Source: CAD feature listing. Evaluate the final solid. Frame: model axes, mm. A direction names the side the tool comes from. Coordinates: 2 decimals unless noted, no trailing zeros. Order: outer loops, then holes, each group sorted by start corner. A loop starts at its lowest first (then second) coordinate and runs counter-clockwise, first axis right, second up. Notation, with made-up numbers: (74.25, 67.25) -> (117.25, 67.25) arc R25 ccw to (117.25, 104.25) -> close; hole circle Ø10 at (34.5, -29.75). An arc over 180 degrees is marked (long way). Write item = value, one per line. Start each with the question number.
Item 1: Mould query, pull axis X, two halves, no side actions, for faces 1 (the cylindrical face through (-0.09, -37.1, 2.03)), 2 (the flat face through (0, 40, 2)), 3 (the flat face through (0, 6.66, 2.92)). Classes: released by +X, released by -X, zero draft, split by the parting line, or undercut.
Item 2: Set-up query: faces 4 (the flat face through (5, -10, 2)), 5 (the flat face through (-5, 1, 0)). Return all of +Z, -Z, +X, -X, +Y, -Y with unobstructed straight access to the full face (end or side cutting, diameter ignored); none if empty.
Item 3: Section query C-C (x = 4.25). Output: boundary loops of the cut face in (y, z), then the cut area to 3 significant figures.
Item 4: Section query B-B (y = 7.3). Output: boundary loops of the cut face in (x, z).
Item 5: Contact query for flat-ended pins moving along their axis: pin 1 (2 mm diameter, centred on y = -7.5, z = 2, fed in from +X); pin 2 (4 mm diameter, centred on x = 0, y = 35, fed in from -Z). Output: stop coordinate, or through.
Item 6: Section query D-D (y = -9). Output: boundary loops of the cut face in (x, z), then the cut area to 3 significant figures.
Item 7: Ray query, line 1 along Z through (x, y) = (-7.5, 7.3); line 2 along X through (y, z) = (-35, 1.55); line 3 along Y through (x, z) = (-5.5, 2.15). Return the intervals inside material, ascending. Write a range as [from, to].
Item 8: Section query A-A (z = 2). Output: boundary loops of the cut face in (x, y).
Solid Edge part; units mm, degrees
sketch "Sketch1" plane through (0, 0, 0) normal (0, 0, 1) x (1, 0, 0)
  line L0 (-10, -40) -> (10, -40)
  line L1 (10, -40) -> (10, 40)
  line L2 (10, 40) -> (-10, 40)
  line L3 (-10, 40) -> (-10, -40)
  circle A0 centre (0, 0) radius 4.6
  dimension "D1" = 10
  dimension "D2" = 10
extrude "Protrusion1" add sketch "Sketch1" along normal blind 4
sketch "Sketch2" plane through (0, 0, 4) normal (0, 0, 1) x (1, 0, 0)
  line L0 (0, 10) -> (10, 10)
  line L1 (10, 10) -> (10, -10)
  line L2 (10, -10) -> (0, -10)
  line L3 (0, -10) -> (0, 10)
  dimension "D1" = 10
extrude "Cutout1" cut sketch "Sketch2" against normal up to next
sketch "Sketch3" plane through (0, 0, 4) normal (0, 0, 1) x (0, 1, 0)
  circle A0 centre (35, 0) radius 2.1
  circle A1 centre (-35, 0) radius 2.1
extrude "Cutout2" cut sketch "Sketch3" against normal up to next
hole "Hole_1" at (0, 7.3, 2) direction (-1, 0, 0) diameter 1.867 depth 10 thread major 2.3 thread length 8
hole "Hole1" at (0, -7.3, 2) direction (-1, 0, 0) diameter 1.867 depth 10 thread major 2.3 thread length 8
Computed:
q1.face_1 = undercut
q1.face_2 = zero draft
q1.face_3 = released by +X
q2.face_4 = +Z, -Z, +X
q2.face_5 = -Z, +X, -X, +Y, -Y
q3.outline = (-40, 0) -> (-10, 0) -> (-10, 4) -> (-40, 4) -> close; (10, 0) -> (40, 0) -> (40, 4) -> (10, 4) -> close
q3.area = 240 mm^2
q4.outline = (-10, 0) -> (0, 0) -> (0, 1.07) -> (-10, 1.07) -> close; (-10, 2.93) -> (0, 2.93) -> (0, 4) -> (-10, 4) -> close
q5.pin_1 = 0
q5.pin_2 = through
q6.outline = (-10, 0) -> (0, 0) -> (0, 4) -> (-10, 4) -> close
q6.area = 40.0 mm^2
q7.line_1 = [0, 1.07], [2.93, 4]
q7.line_2 = [-10, -2.1], [2.1, 10]
q7.line_3 = [-40, -8.22], [-6.38, 6.38], [8.22, 40]
q8.outline = (-10, -40) -> (10, -40) -> (10, -10) -> (0, -10) -> (0, -8.23) -> (-10, -8.23) -> close; (-10, -6.37) -> (0, -6.37) -> (0, -4.6) arc R4.6 cw to (0, 4.6) -> (0, 6.37) -> (-10, 6.37) -> close; (-10, 8.23) -> (0, 8.23) -> (0, 10) -> (10, 10) -> (10, 40) -> (-10, 40) -> close; hole circle Ø4.2 at (0, -35); hole circle Ø4.2 at (0, 35)
